The listing builds one solid part. Answer for the finished solid, in the listing's coordinates (mm). A direction names the side the tool comes from. Coordinates: 2 decimals unless noted, no trailing zeros. Write each loop counter-clockwise with the first axis right and the second up, starting at its lowest first coordinate (ties: lowest second). Pieces come first, ordered by that corner, then holes.
```python
from build123d import *

# Parameters (mm, degrees)
F0_W           = 50.8
F0_H           = 50.8
F1_DEPTH       = 56.45
F2_W           = 44.45
F2_H           = 44.45
F3_DEPTH       = 28
F5_D           = 11
F5_CBORE_D     = 17.25
F5_CBORE_DEPTH = 10
F6_SIZE2       = 11.849251
F6_SIZE        = 3.17499
F8_W           = 4.7625
F8_H           = 20.6375
F9_DEPTH       = 50.801


# Not quite as in the source:
# - a fillet or chamfer is up to 0.001 mm smaller than in the source, because OpenCascade refuses the exact size


with BuildPart() as f1:
    # F0 (on Top) → F1 (new body)
    with BuildSketch(Plane.XY):
        Rectangle(F0_W, F0_H)
    extrude(amount=F1_DEPTH)

    # F2 (on face) → F3 (cut)
    with BuildSketch(Plane.XY.offset(56.45)):
        Rectangle(F2_W, F2_H)
    extrude(amount=-F3_DEPTH, mode=Mode.SUBTRACT)

    # F5 (through all)
    with Locations(Plane.XY.offset(28.45)):
        with Locations((0, 0)):
            CounterBoreHole(F5_D / 2, F5_CBORE_D / 2, F5_CBORE_DEPTH)

    # F6 (size 3.175 and 11.849261314 in the source; OpenCascade refuses exactly that, so slightly less here)
    f6_edges = [f1.edges().sort_by_distance(p)[0] for p in [
        (0, 25.4, 56.45),
        (25.4, 0, 56.45),
        (0, -25.4, 56.45),
        (-25.4, 0, 56.45),
    ]]
    f6_side = f1.faces().sort_by_distance((0, -24.68158, 56.45))[0]
    chamfer(f6_edges, length=F6_SIZE, length2=F6_SIZE2, reference=f6_side)

    # F8 (on offset) → F9 (cut, through all)
    with BuildSketch(Plane(origin=(0, 25.4, 0), x_dir=(-1, 0, 0), z_dir=(0, 1, 0))):
        with BuildLine():
            ThreePointArc((-2.38125, 32.41875), (0, 30.0375), (2.38125, 32.41875))
            Line((2.38125, 32.41875), (-2.38125, 32.41875))
        make_face()
        with Locations((0, 42.7375)):
            Rectangle(F8_W, F8_H)
        with BuildLine():
            Line((-2.38125, 53.05625), (2.38125, 53.05625))
            ThreePointArc((2.38125, 53.05625), (0, 55.4375), (-2.38125, 53.05625))
        make_face()
    extrude(amount=-F9_DEPTH, mode=Mode.SUBTRACT)


solid = f1.part
```
(1) For a pull along Y with two mould halves and no side action, classify faces 4 (the flat face through (0, 6, 0)), 5 (the flat face through (10, 0, 28.45)), 6 (the flat face through (0, 25.4, 22)) as pulls with the +Y half, pulls with the -Y half, needs draft (parallel to the pull), parting line crosses it, or undercut.
(2) Section B-B, the plane z = 38.5 is taken. Write down the section's boundary in (x, y) (3 decimals).
(3) Which of the six approach directions +Z, -Z, +X, -X, +Y, -Y give full straight-line access (tool end or side, diameter ignored) to faces 1 (the flat face through (2.381, -24, 40)), 2 (the flat face through (5.289, -23.835, 50.442)), 3 (the flat face through (-22.225, 0, 43))?
(4) Section D-D, the plane z = 16.5 is taken. Write down the section's boundary in (x, y).
(5) Section C-C, the plane x = 0 is taken. State how many separate pieces and enclosed holes the cut face has, plus the area to 3 significant figures.
(6) Each of these flat-tipped pins is pushed along its axis until it touches: pin 1 (4 mm diameter, centred on x = 6.5, y = -8.5, fed in from +Z); pin 2 (12.5 mm diameter, centred on x = 0, y = 0, fed in from +Z); pin 3 (1 mm diameter, centred on y = 24.5, z = 45.5, fed in from -X). Where does it stop, or does it pass through?
(7) Find the intervals of material crossed by probe 1 along Y at (x, z) = (12, 38) (3 decimals); probe 2 along Y at (x, z) = (0, 22.75) (3 decimals), in increasing order.
Solution:
1. face 4: needs draft
1. face 5: undercut
1. face 6: pulls with the +Y half
2. outline: (-25.4, -25.4) - (-2.381, -25.4) - (-2.381, -22.225) - (-22.225, -22.225) - (-22.225, 22.225) - (-2.381, 22.225) - (-2.381, 25.4) - (-25.4, 25.4) - close; (2.381, -25.4) - (25.4, -25.4) - (25.4, 25.4) - (2.381, 25.4) - (2.381, 22.225) - (22.225, 22.225) - (22.225, -22.225) - (2.381, -22.225) - close
3. face 1: +Y, -Y
3. face 2: +Z, +X, -X, -Y
3. face 3: +Z
4. outline: (-25.4, -25.4) - (25.4, -25.4) - (25.4, 25.4) - (-25.4, 25.4) - close; hole circle Ø11 at (0, 0)
5. separate pieces: 4
5. enclosed holes: 0
5. area: 1,080 mm2
6. pin 1: stops at z = 28.45
6. pin 2: stops at z = 18.45
6. pin 3: stops at x = -25.29
7. probe 1: y = -25.4 to -22.225, 22.225 to 25.4
7. probe 2: y = -25.4 to -8.625, 8.625 to 25.4
